Source: CAD feature listing. Evaluate the final solid. Frame: model axes, mm. Round coordinates to 2 decimals unless told otherwise and drop trailing zeros. Loops run counter-clockwise (first coordinate to the right, second up) from the corner with the lowest first, then second, coordinate; pieces in that order, holes last. Notation, with made-up numbers: M -13,68 L -7,68 A22 ccw -7,86 Z; hole C -16.75,-17 d7. An arc over 180 degrees is marked long. Write each question's results on one line, items separated by ' | '. Start each with the question number.
1. Ray query, line 1 (Z direction, x = 23.25, y = 16); line 2 (Y direction, x = 12, z = 404) (3 decimals); line 3 (X direction, y = 29, z = 128.5) (3 decimals). Return the intervals inside material, ascending.
2. Section A-A on x = 6.5. Output: boundary loops of the cut face in (y, z) (3 decimals).
3. Section B-B on z = 615. Output: boundary loops of the cut face in (x, y) (3 decimals).
4. Contact query for a flat-ended pin moving along its axis: pin 1 Ø7 at (y, z) = (16, 213.6) entering from -X (3 decimals). Output: stop coordinate, or through.
5. Section C-C on z = 386. Output: boundary loops of the cut face in (x, y) (3 decimals), and give its area (3 significant figures).
from build123d import *

# Parameters (mm, degrees)
F0_W     = 50.8
F0_H     = 76.2
F0_W_2   = 44.45
F0_H_2   = 69.85
F2_DEPTH = 762
F3_R     = 3.175
F4_R     = 3
F5_DEPTH = 50.801
F6_W     = 69.85
F6_H     = 379.5014
F6_R     = 3
F7_DEPTH = 25.4


# Not quite as in the source:
# - a variable given as a bare number and used for a length is read in inches; the dataset says mm whatever the document's units were


with BuildPart() as f2:
    # F0 (on Top) → F2 (new body)
    with BuildSketch(Plane.XY):
        Rectangle(F0_W, F0_H)
        Rectangle(F0_W_2, F0_H_2, mode=Mode.SUBTRACT)
    extrude(amount=F2_DEPTH)

    # F3
    f3_edges = [f2.edges().sort_by_distance(p)[0] for p in [
        (-22.225, 34.925, 381),
        (22.225, 34.925, 381),
        (22.225, -34.925, 381),
        (-22.225, -34.925, 381),
        (25.4, 38.1, 381),
        (-25.4, 38.1, 381),
        (25.4, -38.1, 381),
        (-25.4, -38.1, 381),
    ]]
    fillet(f3_edges, radius=F3_R)

    # F4 (on face) → F5 (cut, through all)
    with BuildSketch(Plane.YZ.offset(25.4)):
        with Locations((-16, 213.6)):
            Circle(F4_R)
        with Locations((-16, 243.6)):
            Circle(F4_R)
        with Locations((16, 243.6)):
            Circle(F4_R)
        with Locations((16, 213.6)):
            Circle(F4_R)
        with Locations((-16, 518.4)):
            Circle(F4_R)
        with Locations((-16, 548.4)):
            Circle(F4_R)
        with Locations((16, 518.4)):
            Circle(F4_R)
        with Locations((16, 548.4)):
            Circle(F4_R)
    extrude(amount=-F5_DEPTH, mode=Mode.SUBTRACT)

    # F6 (on face) → F7 (cut)
    with BuildSketch(Plane(origin=(-25.4, 0, 0), x_dir=(0, -1, 0), z_dir=(-1, 0, 0))):
        with Locations((0, 382.9008626968)):
            Rectangle(F6_W, F6_H)
        with Locations((-16, 213.6)):
            Circle(F6_R, mode=Mode.SUBTRACT)
        with Locations((-16, 243.6)):
            Circle(F6_R, mode=Mode.SUBTRACT)
        with Locations((16, 213.6)):
            Circle(F6_R, mode=Mode.SUBTRACT)
        with Locations((16, 243.6)):
            Circle(F6_R, mode=Mode.SUBTRACT)
        with Locations((-16, 518.4)):
            Circle(F6_R, mode=Mode.SUBTRACT)
        with Locations((-16, 548.4)):
            Circle(F6_R, mode=Mode.SUBTRACT)
        with Locations((16, 518.4)):
            Circle(F6_R, mode=Mode.SUBTRACT)
        with Locations((16, 548.4)):
            Circle(F6_R, mode=Mode.SUBTRACT)
    extrude(amount=-F7_DEPTH, mode=Mode.SUBTRACT)


solid = f2.part
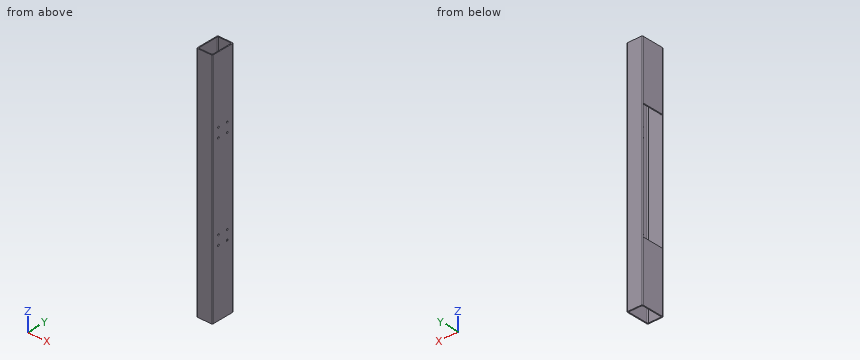
Taken from the geometry:
1) line 1: 0 to 210.6, 216.6 to 240.6, 246.6 to 515.4, 521.4 to 545.4, 551.4 to 762 | line 2: -38.1 to -34.925, 34.925 to 38.1 | line 3: -25.4 to -22.225, 22.225 to 25.4
2) outline: M -38.1,0 L -34.925,0 L -34.925,762 L -38.1,762 Z; M 34.925,0 L 38.1,0 L 38.1,762 L 34.925,762 Z
3) outline: M -25.4,-34.925 A3.175 ccw -22.225,-38.1 L 22.225,-38.1 A3.175 ccw 25.4,-34.925 L 25.4,34.925 A3.175 ccw 22.225,38.1 L -22.225,38.1 A3.175 ccw -25.4,34.925 Z; hole M -22.225,-31.75 A3.175 ccw -19.05,-34.925 L 19.05,-34.925 A3.175 ccw 22.225,-31.75 L 22.225,31.75 A3.175 ccw 19.05,34.925 L -19.05,34.925 A3.175 ccw -22.225,31.75 Z
4) pin 1: x = 22.225
5) outline: M -25.4,-34.925 A3.175 ccw -22.225,-38.1 L 22.225,-38.1 A3.175 ccw 25.4,-34.925 L 25.4,34.925 A3.175 ccw 22.225,38.1 L -22.225,38.1 A3.175 ccw -25.4,34.925 L 19.05,34.925 A3.175 cw 22.225,31.75 L 22.225,-31.75 A3.175 cw 19.05,-34.925 Z | area: 540 mm^2
